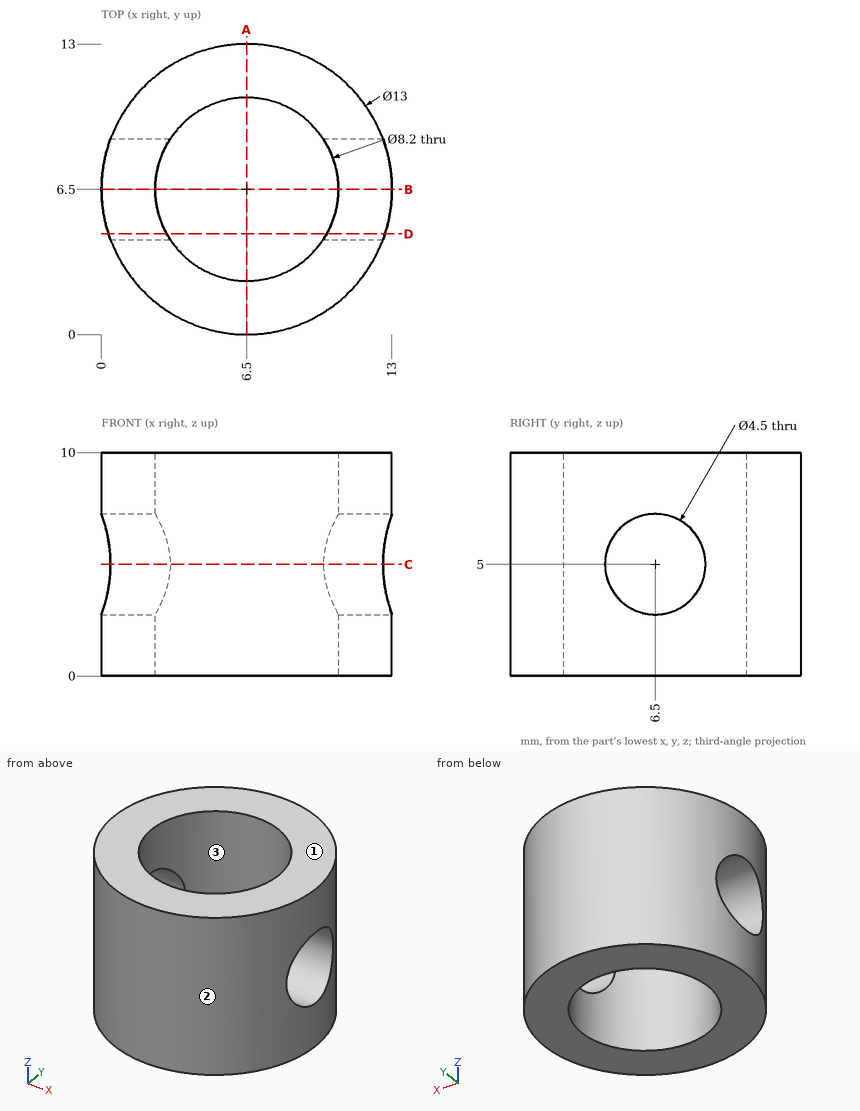
Drawing for the job (mm, zero at the part's lowest x, y, z). Coordinates: 2 decimals unless noted, no trailing zeros. Order: outer loops, then holes, each group sorted by start corner. A loop starts at its lowest first (then second) coordinate and runs counter-clockwise, first axis right, second up.
Item 1: Band-saw the part on A-A on x = 6.5. List the corners of the cut face in (y, z), plus the area to 3 significant figures.
Check sheet entries:
outline: (0, 0) - (2.4, 0) - (2.4, 10) - (0, 10) - close; (10.6, 0) - (13, 0) - (13, 10) - (10.6, 10) - close
area: 48.0 mm2
Item 2: Two-plate mould, pull along X, no slides. Class the marked faces 1, 2 and 3: +X half, -X half, draft (parallel to the pull), parting line (faces both ways), or undercut.
Check sheet entries:
face 1: draft
face 2: parting line
face 3: undercut
Item 3: Drill centre lines: L1, parallel to Y at x = 6.5, z = 4.75; L2, parallel to Y at x = 5, z = 6.25; L3, parallel to X at y = 3.25, z = 3. Where is each one in solid material? Low to high.
Check sheet entries:
L1: y = 0 to 2.4, 10.6 to 13
L2: y = 0.18 to 2.68, 10.32 to 12.82
L3: x = 0.87 to 4, 9 to 12.13
Item 4: Band-saw the part on D-D on y = 4.5. List the corners of the cut face in (x, z).
Check sheet entries:
outline: (0.32, 0) - (2.92, 0) - (2.92, 3.97) - (0.32, 3.97) - close; (0.32, 6.03) - (2.92, 6.03) - (2.92, 10) - (0.32, 10) - close; (10.08, 0) - (12.68, 0) - (12.68, 3.97) - (10.08, 3.97) - close; (10.08, 6.03) - (12.68, 6.03) - (12.68, 10) - (10.08, 10) - close
Item 5: Band-saw the part on B-B on y = 6.5. List the corners of the cut face in (x, z).
Check sheet entries:
outline: (0, 0) - (2.4, 0) - (2.4, 2.75) - (0, 2.75) - close; (0, 7.25) - (2.4, 7.25) - (2.4, 10) - (0, 10) - close; (10.6, 0) - (13, 0) - (13, 2.75) - (10.6, 2.75) - close; (10.6, 7.25) - (13, 7.25) - (13, 10) - (10.6, 10) - close
Item 6: Band-saw the part on C-C on z = 5. List the corners of the cut face in (x, y), plus the area to 3 significant figures.
Check sheet entries:
outline: (0.4, 4.25) arc R6.5 ccw to (12.6, 4.25) - (9.93, 4.25) arc R4.1 cw to (3.07, 4.25) - close; (0.4, 8.75) - (3.07, 8.75) arc R4.1 cw to (9.93, 8.75) - (12.6, 8.75) arc R6.5 ccw to start
area: 57.6 mm2
Item 7: Pin check, flat tips, straight feed: pin 1 Ø6 at (x, z) = (10.5, 9) entering from -Y; pin 2 Ø6 at (y, z) = (11.5, 1) entering from +X; pin 3 Ø5 at (x, y) = (6.5, 6.5) entering from +Z; pin 4 Ø3 at (y, z) = (2, 3.5) entering from +X. Stop position of each tip, or through.
Check sheet entries:
pin 1: stops at y = 0.08
pin 2: stops at x = 12.68
pin 3: passes through
pin 4: stops at x = 12.27
